```python
from build123d import *

# Parameters (mm, degrees)
SM_BASE_FLANGE_1_DEPTH = 50
SKETCH_6_R             = 6.5
CUT_EXTRUDE_1_DEPTH    = 10
SKETCH_7_R             = 6.5
CUT_EXTRUDE_2_DEPTH    = 10
OTHER_START            = 147.502474556
OTHER_1_OUTLINE_W      = 10
OTHER_1_OUTLINE_H      = 8
OTHER_1_DEPTH          = 3.535533905
OTHER_START_2          = 182.857813615
OTHER_1_2_OUTLINE_W    = 38
OTHER_1_2_OUTLINE_H    = 8
OTHER_1_2_DEPTH        = 3.535533906
OTHER_1_3_OUTLINE_W    = 7
OTHER_1_3_OUTLINE_H    = 10
OTHER_1_3_DEPTH        = 3.535533906
OTHER_START_3          = -35.355339059
OTHER_1_4_OUTLINE_W    = 7
OTHER_1_4_OUTLINE_H    = 38
OTHER_1_4_DEPTH        = 3.535533906


# Read off the part's stored shape, not the designer's step: Затупленный угол1
# Sheet-metal steps are written as plain solids
with BuildPart() as part:
    # Sketch 1 → Базовая кромка1 (new body)
    with BuildSketch(Plane.XY):
        with BuildLine():
            Line((213.6, 404.5), (163.6, 404.5))
            ThreePointArc((163.6, 404.5), (156.528932188, 401.571067812), (153.6, 394.5))
            Line((153.6, 394.5), (153.6, 350.548284888))
            ThreePointArc((153.6, 350.548284888), (152.511654958, 344.938841391), (149.404552488, 340.143399231))
            Line((149.404552488, 340.143399231), (2.796965008, 187.904400513))
            ThreePointArc((2.796965008, 187.904400513), (0.725563362, 184.707439072), (0, 180.967810075))
            Line((0, 180.967810075), (0, 0))
            Line((0, 0), (-5, 0))
            Line((-5, 0), (-5, 180.967810075))
            ThreePointArc((-5, 180.967810075), (-3.911654958, 186.577253571), (-0.804552488, 191.372695731))
            Line((-0.804552488, 191.372695731), (145.803034992, 343.61169445))
            ThreePointArc((145.803034992, 343.61169445), (147.874436638, 346.80865589), (148.6, 350.548284888))
            Line((148.6, 350.548284888), (148.6, 394.5))
            ThreePointArc((148.6, 394.5), (152.993398282, 405.106601718), (163.6, 409.5))
            Line((163.6, 409.5), (213.6, 409.5))
            Line((213.6, 409.5), (213.6, 404.5))
        make_face()
    extrude(amount=SM_BASE_FLANGE_1_DEPTH)

    # Эскиз6 → Вырез-Вытянуть1 (cut)
    with BuildSketch(Plane.ZY.offset(5)):
        with Locations(Location((15, 15, 0), (0, 0, 270))):
            Circle(SKETCH_6_R)
        with Locations(Location((15, 40, 0), (0, 0, 270))):
            Circle(SKETCH_6_R)
    extrude(amount=-CUT_EXTRUDE_1_DEPTH, mode=Mode.SUBTRACT)

    # Эскиз7 → Вырез-Вытянуть2 (cut)
    with BuildSketch(Plane(origin=(0, 409.5, 0), x_dir=(1, 0, 0), z_dir=(0, 1, 0))):
        with Locations(Location((188.6, -25, 0), (0, 0, 180))):
            Circle(SKETCH_7_R)
    extrude(amount=-CUT_EXTRUDE_2_DEPTH, mode=Mode.SUBTRACT)

    # Other 1 outline → Other 1 (cut)
    with BuildSketch(Plane(origin=(0, 0, 0), x_dir=(0.707106781186548, 0, 0.707106781186547), z_dir=(0.707106781186547, 0, -0.707106781186548)).offset(OTHER_START)):
        with Locations((151, -407)):
            Rectangle(OTHER_1_OUTLINE_W, OTHER_1_OUTLINE_H)
    extrude(amount=OTHER_1_DEPTH, mode=Mode.SUBTRACT)

    # Other 1 2 outline → Other 1 2 (cut)
    with BuildSketch(Plane(origin=(0, 0, 0), x_dir=(0.707106781186548, 0, -0.707106781186547), z_dir=(0.707106781186547, 0, 0.707106781186548)).offset(OTHER_START_2)):
        with Locations((130, 407)):
            Rectangle(OTHER_1_2_OUTLINE_W, OTHER_1_2_OUTLINE_H)
    extrude(amount=OTHER_1_2_DEPTH, mode=Mode.SUBTRACT)

    # Other 1 3 outline → Other 1 3 (cut)
    with BuildSketch(Plane(origin=(0, 0, 0), x_dir=(1, 0, 0), z_dir=(0, 0.707106781186547, 0.707106781186548))):
        with Locations((-2.5, 0)):
            Rectangle(OTHER_1_3_OUTLINE_W, OTHER_1_3_OUTLINE_H)
    extrude(amount=OTHER_1_3_DEPTH, mode=Mode.SUBTRACT)

    # Other 1 4 outline → Other 1 4 (cut)
    with BuildSketch(Plane(origin=(0, 0, 0), x_dir=(1, 0, 0), z_dir=(0, 0.707106781186547, -0.707106781186548)).offset(OTHER_START_3)):
        with Locations((-2.5, -21)):
            Rectangle(OTHER_1_4_OUTLINE_W, OTHER_1_4_OUTLINE_H)
    extrude(amount=OTHER_1_4_DEPTH, mode=Mode.SUBTRACT)


solid = part.part
```
Geometry: final body of the model. Coordinates: model frame, mm. A direction names the side the tool comes from. Round coordinates to 2 decimals unless told otherwise and drop trailing zeros. Order: outer loops, then holes, each group sorted by start corner. A loop starts at its lowest first (then second) coordinate and runs counter-clockwise, first axis right, second up. Notation, with made-up numbers: M -22.5,0 L -7.5,0 A29 ccw -7.5,20 Z; hole C 48,9 d6. An arc over 180 degrees is marked long. Use one line per item in the form item = value. Start each with the question number.
Q1. Pin query (flat end, axial travel): pin 1 Ø22 at (y, z) = (376.5, 32) entering from -X; pin 2 Ø8 at (y, z) = (304.5, 5.5) entering from +X; pin 3 Ø2 at (y, z) = (198.5, 40) entering from +X; pin 4 Ø8 at (y, z) = (15, 15) entering from -X. Return the tip coordinate at first contact, or that it passes through.
Q2. Mould query, pull axis Y, two halves, no side actions, for faces 1 (the face through (-2.535, 46.494, 15.286)), 2 (the face through (-2.535, 21.494, 15.286)), 3 (the face through (0, 92, 25)), 4 (the face through (183, 409.5, 19)). Classes: +Y half, -Y half, draft (parallel to the pull), parting line (faces both ways), or undercut.
Q3. Access query for faces 5 (the face through (182.4, 407.04, 26.95)), 6 (the face through (153.6, 373, 25)), 7 (the face through (148.6, 372, 25)). Directions: +Z, -Z, +X, -X, +Y, -Y. A direction counts if a zero-diameter tool reaches every point of the face in a straight line with its end or side. Return the directions, or none.
Q4. Cut plane D-D (x = 129.5). Return loops of the section in (y, z).
Q5. Cut plane C-C (y = 375). Return loops of the section in (x, z), and give its area (3 significant figures).
Q6. Cut plane B-B (x = 187.5). Return loops of the section in (y, z).
Q7. Cut plane A-A (y = 15). Return loops of the section in (x, z), and give its area (3 significant figures).
Q8. Material intervals for line 1 (Z direction, x = -3, y = 15); line 2 (Z direction, x = 188.6, y = 407.95); line 3 (X direction, y = 23.5, z = 25), sorted ascending. Write a range as [from, to].
Geometry results:
q1.pin_1 = 148.6
q1.pin_2 = 118.93
q1.pin_3 = 13.96
q1.pin_4 = through
q2.face_1 = undercut
q2.face_2 = undercut
q2.face_3 = draft
q2.face_4 = +Y half
q3.face_5 = +Y, -Y
q3.face_6 = +Z, -Z, +X, -Y
q3.face_7 = +Z, -Z, -X, +Y
q4.outline = M 319.47,0 L 326.68,0 L 326.68,50 L 319.47,50 Z
q5.outline = M 148.6,0 L 153.6,0 L 153.6,50 L 148.6,50 Z
q5.area = 250 mm^2
q6.outline = M 404.5,0 L 409.5,0 L 409.5,18.59 L 404.5,18.59 Z; M 404.5,31.41 L 409.5,31.41 L 409.5,50 L 404.5,50 Z
q7.outline = M -5,0 L 0,0 L 0,8.5 L -5,8.5 Z; M -5,21.5 L 0,21.5 L 0,50 L -5,50 Z
q7.area = 185 mm^2
q8.line_1 = [0, 8.5], [21.5, 50]
q8.line_2 = [0, 18.5], [31.5, 50]
q8.line_3 = [-5, 0]
